Read the model definition and answer for the solid it produces. Units are mm, in the model's axes. A direction names the side the tool comes from. Give positions to 0.01 mm unless a question says otherwise; leave off trailing zeros. Write each loop counter-clockwise with the first axis right and the second up, starting at its lowest first coordinate (ties: lowest second). Pieces come first, ordered by that corner, then holes.
```python
from build123d import *

# Parameters (mm, degrees)
SKETCH2_W           = 42
SKETCH2_H           = 42
SKETCH2_R           = 5.5
BOSS_EXTRUDE1_DEPTH = 2
SKETCH4_W           = 42
SKETCH4_H           = 42
BOSS_EXTRUDE2_DEPTH = 3
BOSS_EXTRUDE3_DEPTH = 3
BOSS_EXTRUDE5_DEPTH = 5
CUT_EXTRUDE1_DEPTH  = 2.5
SKETCH9_R           = 1.35
CUT_EXTRUDE2_DEPTH  = 8
FILLET1_R           = 3
FILLET2_R           = 1
CHAMFER1_SIZE       = 0.5
SKETCH11_W          = 17.78
SKETCH11_H          = 17.5
CUT_EXTRUDE3_DEPTH  = 7
FILLET3_R           = 2
FILLET4_R           = 0.5


with BuildPart() as part:
    # Sketch2 → Boss-Extrude1 (new body)
    with BuildSketch(Plane(origin=(0, 0, 0), x_dir=(1, 0, 0), z_dir=(0, 1, 0))):
        Rectangle(SKETCH2_W, SKETCH2_H)
        with Locations((0, 6)):
            Circle(SKETCH2_R, mode=Mode.SUBTRACT)
    extrude(amount=-BOSS_EXTRUDE1_DEPTH)

    # Sketch4 → Boss-Extrude2 (add)
    with BuildSketch(Plane.XZ.offset(2)):
        Rectangle(SKETCH4_W, SKETCH4_H)
        with BuildLine():
            Line((-17, 11.522774425), (-17, -11.522774425))
            ThreePointArc((-17, -11.522774425), (-16.869274473, -11.859874356), (-16.545454545, -12.020704023))
            ThreePointArc((-16.545454545, -12.020704023), (-13.464466094, -13.464466094), (-12.020704023, -16.545454545))
            ThreePointArc((-12.020704023, -16.545454545), (-11.859874356, -16.869274473), (-11.522774425, -17))
            Line((-11.522774425, -17), (11.522774425, -17))
            ThreePointArc((11.522774425, -17), (11.859874356, -16.869274473), (12.020704023, -16.545454545))
            ThreePointArc((12.020704023, -16.545454545), (13.464466094, -13.464466094), (16.545454545, -12.020704023))
            ThreePointArc((16.545454545, -12.020704023), (16.869274473, -11.859874356), (17, -11.522774425))
            Line((17, -11.522774425), (17, 11.522774425))
            ThreePointArc((17, 11.522774425), (16.869274473, 11.859874356), (16.545454545, 12.020704023))
            ThreePointArc((16.545454545, 12.020704023), (13.464466094, 13.464466094), (12.020704023, 16.545454545))
            ThreePointArc((12.020704023, 16.545454545), (11.859874356, 16.869274473), (11.522774425, 17))
            Line((11.522774425, 17), (-11.522774425, 17))
            ThreePointArc((-11.522774425, 17), (-11.859874356, 16.869274473), (-12.020704023, 16.545454545))
            ThreePointArc((-12.020704023, 16.545454545), (-13.464466094, 13.464466094), (-16.545454545, 12.020704023))
            ThreePointArc((-16.545454545, 12.020704023), (-16.869274473, 11.859874356), (-17, 11.522774425))
        make_face(mode=Mode.SUBTRACT)
    extrude(amount=BOSS_EXTRUDE2_DEPTH)

    # Sketch6 → Boss-Extrude3 (add)
    with BuildSketch(Plane.XZ.offset(2)):
        with BuildLine():
            Line((-17, 11.522774425), (-17, -11.522774425))
            ThreePointArc((-17, -11.522774425), (-16.869274473, -11.859874356), (-16.545454545, -12.020704023))
            ThreePointArc((-16.545454545, -12.020704023), (-13.464466094, -13.464466094), (-12.020704023, -16.545454545))
            ThreePointArc((-12.020704023, -16.545454545), (-11.859874356, -16.869274473), (-11.522774425, -17))
            Line((-11.522774425, -17), (11.522774425, -17))
            ThreePointArc((11.522774425, -17), (11.859874356, -16.869274473), (12.020704023, -16.545454545))
            ThreePointArc((12.020704023, -16.545454545), (13.464466094, -13.464466094), (16.545454545, -12.020704023))
            ThreePointArc((16.545454545, -12.020704023), (16.869274473, -11.859874356), (17, -11.522774425))
            Line((17, -11.522774425), (17, 11.522774425))
            ThreePointArc((17, 11.522774425), (16.869274473, 11.859874356), (16.545454545, 12.020704023))
            ThreePointArc((16.545454545, 12.020704023), (13.464466094, 13.464466094), (12.020704023, 16.545454545))
            ThreePointArc((12.020704023, 16.545454545), (11.859874356, 16.869274473), (11.522774425, 17))
            Line((11.522774425, 17), (-11.522774425, 17))
            ThreePointArc((-11.522774425, 17), (-11.859874356, 16.869274473), (-12.020704023, 16.545454545))
            ThreePointArc((-12.020704023, 16.545454545), (-13.464466094, 13.464466094), (-16.545454545, 12.020704023))
            ThreePointArc((-16.545454545, 12.020704023), (-16.869274473, 11.859874356), (-17, 11.522774425))
        make_face()
        with BuildLine():
            Line((-16.5, 11.522774425), (-16.5, -11.522774425))
            ThreePointArc((-16.5, -11.522774425), (-13.110912703, -13.110912703), (-11.522774425, -16.5))
            Line((-11.522774425, -16.5), (11.522774425, -16.5))
            ThreePointArc((11.522774425, -16.5), (13.110912703, -13.110912703), (16.5, -11.522774425))
            Line((16.5, -11.522774425), (16.5, 11.522774425))
            ThreePointArc((16.5, 11.522774425), (13.110912703, 13.110912703), (11.522774425, 16.5))
            Line((11.522774425, 16.5), (-11.522774425, 16.5))
            ThreePointArc((-11.522774425, 16.5), (-13.110912703, 13.110912703), (-16.5, 11.522774425))
        make_face(mode=Mode.SUBTRACT)
    extrude(amount=BOSS_EXTRUDE3_DEPTH)

    # Sketch7 → Boss-Extrude5 (add)
    with BuildSketch(Plane.XZ.offset(2)):
        with BuildLine():
            Line((11.522774425, 16.5), (-11.522774425, 16.5))
            ThreePointArc((-11.522774425, 16.5), (-13.110912703, 13.110912703), (-16.5, 11.522774425))
            Line((-16.5, 11.522774425), (-16.5, -11.522774425))
            ThreePointArc((-16.5, -11.522774425), (-13.110912703, -13.110912703), (-11.522774425, -16.5))
            Line((-11.522774425, -16.5), (11.522774425, -16.5))
            ThreePointArc((11.522774425, -16.5), (13.110912703, -13.110912703), (16.5, -11.522774425))
            Line((16.5, -11.522774425), (16.5, 11.522774425))
            ThreePointArc((16.5, 11.522774425), (13.110912703, 13.110912703), (11.522774425, 16.5))
        make_face()
        with BuildLine():
            Line((10.67544468, 15.5), (-10.67544468, 15.5))
            ThreePointArc((-10.67544468, 15.5), (-12.403805922, 12.403805922), (-15.5, 10.67544468))
            Line((-15.5, 10.67544468), (-15.5, -10.67544468))
            ThreePointArc((-15.5, -10.67544468), (-12.403805922, -12.403805922), (-10.67544468, -15.5))
            Line((-10.67544468, -15.5), (10.67544468, -15.5))
            ThreePointArc((10.67544468, -15.5), (12.403805922, -12.403805922), (15.5, -10.67544468))
            Line((15.5, -10.67544468), (15.5, 10.67544468))
            ThreePointArc((15.5, 10.67544468), (12.403805922, 12.403805922), (10.67544468, 15.5))
        make_face(mode=Mode.SUBTRACT)
    extrude(amount=BOSS_EXTRUDE5_DEPTH)

    # Sketch8 → Cut-Extrude1 (cut)
    with BuildSketch(Plane(origin=(0, 0, 0), x_dir=(1, 0, 0), z_dir=(0, 1, 0))):
        with BuildLine():
            Line((-17, 13), (-21, 13))
            Line((-21, 13), (-21, 21))
            Line((-21, 21), (-13, 21))
            Line((-13, 21), (-13, 17))
            ThreePointArc((-13, 17), (-14.171572875, 14.171572875), (-17, 13))
        make_face()
        with BuildLine():
            Line((13, 17), (13, 21))
            Line((13, 21), (21, 21))
            Line((21, 21), (21, 13))
            Line((21, 13), (17, 13))
            ThreePointArc((17, 13), (14.171572875, 14.171572875), (13, 17))
        make_face()
        with BuildLine():
            Line((-21, -17), (-21, -21))
            Line((-21, -21), (-17, -21))
            Line((-17, -21), (-13, -21))
            Line((-13, -21), (-13, -17))
            ThreePointArc((-13, -17), (-14.171572875, -14.171572875), (-17, -13))
            Line((-17, -13), (-21, -13))
            Line((-21, -13), (-21, -17))
        make_face()
        with BuildLine():
            Line((17, -13), (21, -13))
            Line((21, -13), (21, -21))
            Line((21, -21), (17, -21))
            Line((17, -21), (13, -21))
            Line((13, -21), (13, -17))
            ThreePointArc((13, -17), (14.171572875, -14.171572875), (17, -13))
        make_face()
    extrude(amount=-CUT_EXTRUDE1_DEPTH, mode=Mode.SUBTRACT)

    # Sketch9 → Cut-Extrude2 (cut, through all)
    with BuildSketch(Plane(origin=(0, 0, 0), x_dir=(1, 0, 0), z_dir=(0, 1, 0))):
        with Locations((-17, 17)):
            Circle(SKETCH9_R)
        with Locations((17, 17)):
            Circle(SKETCH9_R)
        with Locations((-17, -17)):
            Circle(SKETCH9_R)
        with Locations((17, -17)):
            Circle(SKETCH9_R)
    extrude(amount=-CUT_EXTRUDE2_DEPTH, mode=Mode.SUBTRACT)

    # Fillet1
    fillet1_edges = [part.edges().sort_by_distance(p)[0] for p in [
        (21, -3.75, 21),
        (-21, -3.75, 21),
        (-21, -3.75, -21),
        (21, -3.75, -21),
    ]]
    fillet(fillet1_edges, radius=FILLET1_R)

    # Fillet2
    fillet2_edges = [part.edges().sort_by_distance(p)[0] for p in [
        (13, -1.25, -21),
        (21, -1.25, -13),
        (-21, -1.25, 13),
        (-13, -1.25, 21),
        (21, -1.25, 13),
        (13, -1.25, 21),
        (-21, -1.25, -13),
        (-13, -1.25, -21),
    ]]
    fillet(fillet2_edges, radius=FILLET2_R)

    # Chamfer1
    chamfer1_edges = [part.edges().sort_by_distance(p)[0] for p in [
        (-5.5, -2, -6),
    ]]
    chamfer(chamfer1_edges, length=CHAMFER1_SIZE)

    # Sketch11 → Cut-Extrude3 (cut)
    with BuildSketch(Plane(origin=(0, 0, 0), x_dir=(1, 0, 0), z_dir=(0, 1, 0))):
        with Locations((0, -12.25)):
            Rectangle(SKETCH11_W, SKETCH11_H)
    extrude(amount=-CUT_EXTRUDE3_DEPTH, mode=Mode.SUBTRACT)

    # Fillet3
    fillet3_edges = [part.edges().sort_by_distance(p)[0] for p in [
        (-8.89, -1, 3.5),
        (8.89, -1, 3.5),
    ]]
    fillet(fillet3_edges, radius=FILLET3_R)

    # Fillet4
    fillet4_edges = [part.edges().sort_by_distance(p)[0] for p in [
        (-8.89, -2.5, 21),
        (8.89, -2.5, 21),
    ]]
    fillet(fillet4_edges, radius=FILLET4_R)


solid = part.part
```
Item 1: Which of the six approach directions +Z, -Z, +X, -X, +Y, -Y give full straight-line access (tool end or side, diameter ignored) to faces 4 (the flat face through (-13, -1, -19)), 5 (the flat face through (-4, -2, 0)), 6 (the cylindrical face through (14.141, -1.232, 14.203))?
Result set:
face 4: -Z, -X, +Y
face 5: -Y
face 6: +Z, +X, +Y
Item 2: Each of these flat-tipped pins is pushed along its axis until it touches: pin 1 Ø2 at (y, z) = (-1, -18.5) entering from -X; pin 2 Ø1.6 at (y, z) = (-6, 2) entering from +X; pin 3 Ø2.5 at (x, z) = (-16.5, -17.5) entering from +Y. Where does it stop, or does it pass through?
Result set:
pin 1: stops at x = -13
pin 2: stops at x = 16.5
pin 3: stops at y = -2.5
Item 3: Find the intervals of material crossed by line 1 along X through (y, z) = (-3.2, -17); line 2 along X through (y, z) = (-3.25, 17); line 3 along X through (y, z) = (-6, 6), in increasing order.
Result set:
line 1: x = -21 to -18.35, -15.65 to 15.65, 18.35 to 21
line 2: x = -21 to -18.35, -15.65 to -8.89, 8.89 to 15.65, 18.35 to 21
line 3: x = -16.5 to -15.5, 15.5 to 16.5
Item 4: Section B-B (z = 6.5) is taken. Write down the section's boundary in (x, y).
Result set:
outline: (-21, -5) - (-16.5, -5) - (-16.5, -7) - (-15.5, -7) - (-15.5, -2) - (-8.89, -2) - (-8.89, 0) - (-21, 0) - close; (8.89, -2) - (15.5, -2) - (15.5, -7) - (16.5, -7) - (16.5, -5) - (21, -5) - (21, 0) - (8.89, 0) - close
Item 5: Section A-A (x = 0) is taken. Write down the section's boundary in (y, z), and give its area (4 significant figures).
Result set:
outline: (-7, -16.5) - (-5, -16.5) - (-5, -21) - (0, -21) - (0, -11.5) - (-1.5, -11.5) - (-2, -12) - (-2, -15.5) - (-7, -15.5) - close; (-2, 0) - (-1.5, -0.5) - (0, -0.5) - (0, 3.5) - (-2, 3.5) - close
area: 45.25 mm2
Item 6: Section D-D (y = -3) is taken. Write down the section's boundary in (x, z), and give its area (3 significant figures).
Result set:
outline: (-21, -18) arc R3 ccw to (-18, -21) - (18, -21) arc R3 ccw to (21, -18) - (21, 18) arc R3 ccw to (18, 21) - (9.39, 21) arc R0.5 ccw to (8.89, 20.5) - (8.89, 15.5) - (10.68, 15.5) arc R6.5 ccw to (15.5, 10.68) - (15.5, -10.68) arc R6.5 ccw to (10.68, -15.5) - (-10.68, -15.5) arc R6.5 ccw to (-15.5, -10.68) - (-15.5, 10.68) arc R6.5 ccw to (-10.68, 15.5) - (-8.89, 15.5) - (-8.89, 20.5) arc R0.5 ccw to (-9.39, 21) - (-18, 21) arc R3 ccw to (-21, 18) - close; hole circle Ø2.7 at (-17, -17); hole circle Ø2.7 at (-17, 17); hole circle Ø2.7 at (17, -17); hole circle Ø2.7 at (17, 17)
area: 739 mm2
Item 7: Determine the mould class of faces 1 (the flat face through (13, -3, 21)), 2 (the cylindrical face through (20.715, -1.268, -12.699)), 3 (the cylindrical face through (15.65, -3.73, -17.06)) for opening direction X: pulls with the +X half, pulls with the -X half, needs draft (parallel to the pull), parting line crosses it, or undercut.
Result set:
face 1: needs draft
face 2: pulls with the +X half
face 3: undercut
